Geometry: see drawing. Coordinates: mm, zero at the bounding-box minimum. Coordinates: 2 decimals unless noted, no trailing zeros. Loops run counter-clockwise (first coordinate to the right, second up) from the corner with the lowest first, then second, coordinate; pieces in that order, holes last. Notation, with made-up numbers: M 21,78.25 L 48,78.25 A19 cw 48,106.25 Z; hole C -20.75,-9.75 d6. An arc over 180 degrees is marked long. Write each question's results on one line, items separated by ' | '. Start each with the question number.
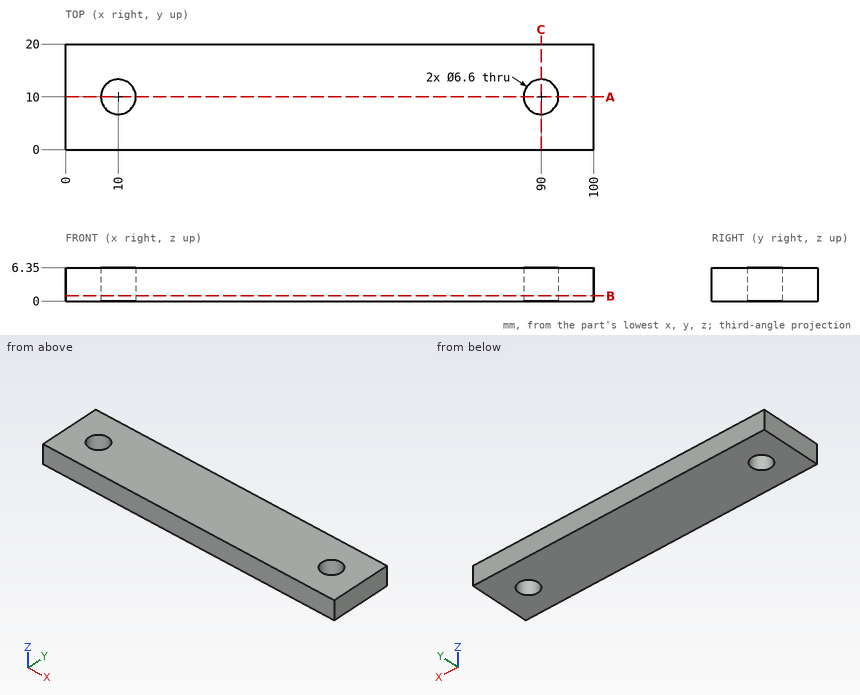
Item 1: First-contact query: pin 1 Ø6 at (x, y) = (90, 10) entering from -Z. Flat tip, straight axial feed; report the tip coordinate or a pass-through.
Item 2: Cut plane C-C (x = 90). Output: boundary loops of the cut face in (y, z).
Item 3: Line query: probe 1 along Y at (x, z) = (10, 5); probe 2 along X at (y, z) = (11.5, 1.5); probe 3 along X at (y, z) = (7.5, 4). Output: solid intervals per line, ascending.
Item 4: Cut plane B-B (z = 1). Output: boundary loops of the cut face in (x, y).
Item 5: Cut plane A-A (y = 10). Output: boundary loops of the cut face in (x, z), then the cut area to 3 significant figures.
Response values:
1) pin 1: passes through
2) outline: M 0,0 L 6.7,0 L 6.7,6.35 L 0,6.35 Z; M 13.3,0 L 20,0 L 20,6.35 L 13.3,6.35 Z
3) probe 1: y = 0 to 6.7, 13.3 to 20 | probe 2: x = 0 to 7.06, 12.94 to 87.06, 92.94 to 100 | probe 3: x = 0 to 7.85, 12.15 to 87.85, 92.15 to 100
4) outline: M 0,0 L 100,0 L 100,20 L 0,20 Z; hole C 10,10 d6.6; hole C 90,10 d6.6
5) outline: M 0,0 L 6.7,0 L 6.7,6.35 L 0,6.35 Z; M 13.3,0 L 86.7,0 L 86.7,6.35 L 13.3,6.35 Z; M 93.3,0 L 100,0 L 100,6.35 L 93.3,6.35 Z | area: 551 mm2
